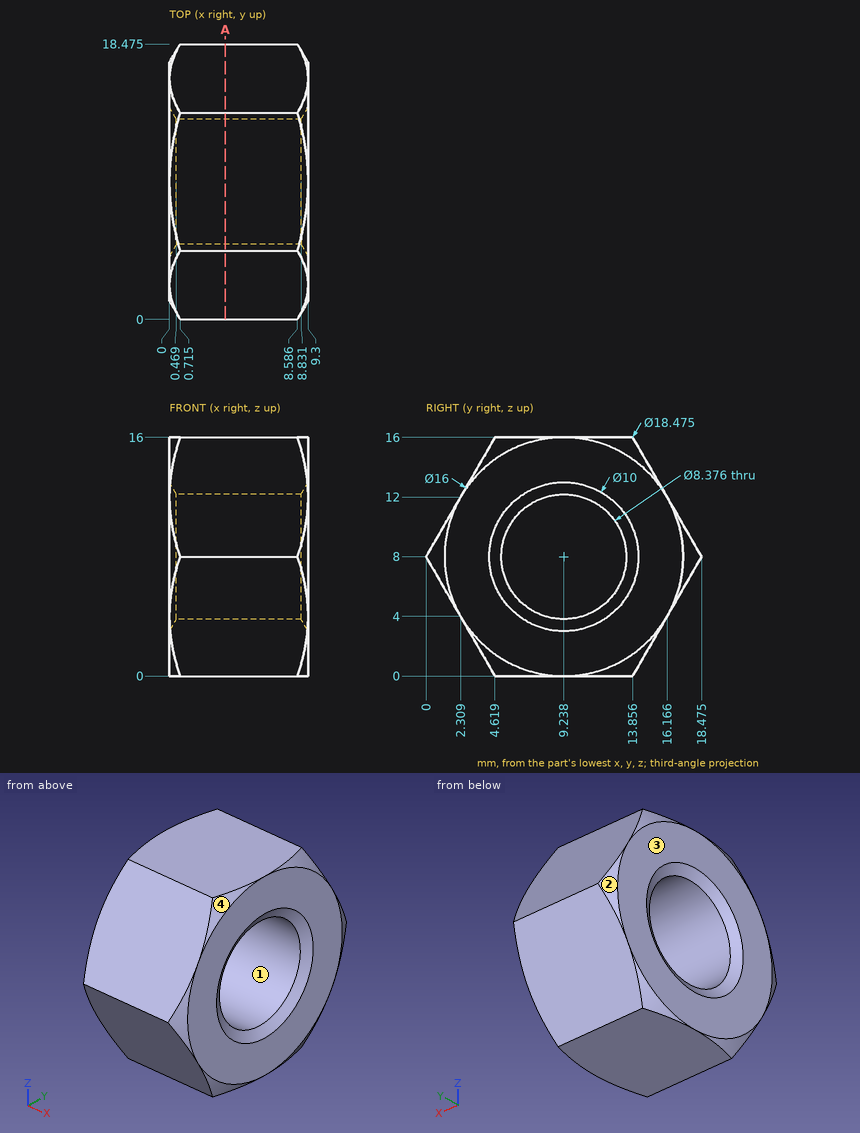
Verification items for this drawing (mm, ordinates from the low corner). Coordinates: 2 decimals unless noted, no trailing zeros. Write each loop counter-clockwise with the first axis right and the second up, starting at its lowest first coordinate (ties: lowest second). Pieces come first, ordered by that corner, then holes. Notation, with made-up numbers: M 28.25,-35 L 87.25,-35 A18 ccw 87.25,-5 Z; hole C 61.25,88 d8. An arc over 180 degrees is marked long. One line per item, written item: value. Start each with the question number.
(1) Depth check by flat-ended pin: pin 1 (5 mm diameter, centred on x = 4, z = 13, fed in from -Y); pin 2 (2 mm diameter, centred on x = 6, z = 10, fed in from -Y); pin 3 (4 mm diameter, centred on x = 1.5, y = 16.5, fed in from -Z) (1 decimal). Enter the tip coordinate at first touch or a pass-through.
(2) Scan lines: line 1 along Z through (x, y) = (7, 8); line 2 along Z through (x, y) = (9, 9) (1 decimal); line 3 along Y through (x, z) = (4, 10) (1 decimal). Record each from-to range of solid material in increasing order. Write a range as [from, to].
(3) Release check for a two-part mould opening along Y. For the marked faces 1, 2, 3 and 4 record: released by +Y, released by -Y, zero draft, split by the parting line, or undercut.
(4) Sectioned sample at A-A, the plane x = 3.75. Enter the section's corners in (y, z) (1 decimal).
Filled sheet:
1. pin 1: y = 1.44
1. pin 2: y = 0.58
1. pin 3: z = 1.1
2. line 1: [0, 4], [12, 16]
2. line 2: [0, 3.5], [12.5, 16]
2. line 3: [1.2, 5.6], [12.9, 17.3]
3. face 1: undercut
3. face 2: released by +Y
3. face 3: zero draft
3. face 4: released by -Y
4. outline: M 0,8 L 4.6,0 L 13.9,0 L 18.5,8 L 13.9,16 L 4.6,16 Z; hole C 9.2,8 d8.4
